from build123d import *

# Parameters (mm, degrees)
SKETCH_R              = 45
PAD_DEPTH             = 20
SKETCH001_R           = 42
POCKET_DEPTH          = 17
POCKET001_DEPTH       = 5
POLARPATTERN_COUNT    = 6
POCKET002_DEPTH       = 5
POLARPATTERN001_COUNT = 6
POCKET003_DEPTH       = 5
POLARPATTERN002_COUNT = 6
POCKET004_DEPTH       = 5
POLARPATTERN003_COUNT = 6
POCKET005_DEPTH       = 5
POLARPATTERN004_COUNT = 6
POCKET006_DEPTH       = 5
CHAMFER_SIZE2         = 2
CHAMFER_SIZE          = 5


with BuildPart() as part:
    # Sketch → Pad (new body)
    with BuildSketch(Plane.XY):
        Circle(SKETCH_R)
    extrude(amount=PAD_DEPTH)

    # Sketch001 (on Face3 of Pad) → Pocket (cut)
    with BuildSketch(Plane.XY.offset(20)):
        Circle(SKETCH001_R)
    extrude(amount=-POCKET_DEPTH, mode=Mode.SUBTRACT)

    # Sketch003 (on Face5 of Pocket) → Pocket001 (cut)
    with BuildSketch(Plane.XY.offset(3)):
        Polygon((-6.25833, 6.5), (-8.75833, 10.830127), (-13.75833, 10.830127), (-16.25833, 6.5), (-13.75833, 2.169873), (-8.75833, 2.169873), align=None)
    pocket001 = extrude(amount=-POCKET001_DEPTH, mode=Mode.SUBTRACT)

    # PolarPattern: Pocket001 ×6 about axis
    polarpattern_axis = Axis((0, 0, 3), (0, 0, 1))
    for i in range(1, POLARPATTERN_COUNT):
        add(pocket001.rotate(polarpattern_axis, i * 360 / POLARPATTERN_COUNT), mode=Mode.SUBTRACT)

    # Sketch004 (on Face41 of PolarPattern) → Pocket002 (cut)
    with BuildSketch(Plane.XY.offset(3)):
        Polygon((13.75833, -23.830127), (16.25833, -19.5), (13.75833, -15.169873), (8.75833, -15.169873), (6.25833, -19.5), (8.75833, -23.830127), align=None)
    pocket002 = extrude(amount=-POCKET002_DEPTH, mode=Mode.SUBTRACT)

    # PolarPattern001: Pocket002 ×6 about axis
    polarpattern001_axis = Axis((0, 0, 3), (0, 0, 1))
    for i in range(1, POLARPATTERN001_COUNT):
        add(pocket002.rotate(polarpattern001_axis, i * 360 / POLARPATTERN001_COUNT), mode=Mode.SUBTRACT)

    # Sketch005 (on Face77 of PolarPattern001) → Pocket003 (cut)
    with BuildSketch(Plane.XY.offset(3)):
        Polygon((2.5, -30.330127), (5, -26), (2.5, -21.669873), (-2.5, -21.669873), (-5, -26), (-2.5, -30.330127), align=None)
    pocket003 = extrude(amount=-POCKET003_DEPTH, mode=Mode.SUBTRACT)

    # PolarPattern002: Pocket003 ×6 about axis
    polarpattern002_axis = Axis((0, 0, 3), (0, 0, 1))
    for i in range(1, POLARPATTERN002_COUNT):
        add(pocket003.rotate(polarpattern002_axis, i * 360 / POLARPATTERN002_COUNT), mode=Mode.SUBTRACT)

    # Sketch006 (on Face113 of PolarPattern002) → Pocket004 (cut)
    with BuildSketch(Plane.XY.offset(3)):
        Polygon((-8.75833, -36.830127), (-6.25833, -32.5), (-8.75833, -28.169873), (-13.75833, -28.169873), (-16.25833, -32.5), (-13.75833, -36.830127), align=None)
    pocket004 = extrude(amount=-POCKET004_DEPTH, mode=Mode.SUBTRACT)

    # PolarPattern003: Pocket004 ×6 about axis
    polarpattern003_axis = Axis((0, 0, 3), (0, 0, 1))
    for i in range(1, POLARPATTERN003_COUNT):
        add(pocket004.rotate(polarpattern003_axis, i * 360 / POLARPATTERN003_COUNT), mode=Mode.SUBTRACT)

    # Sketch007 (on Face149 of PolarPattern003) → Pocket005 (cut)
    with BuildSketch(Plane.XY.offset(3)):
        Polygon((13.75833, -36.830127), (16.25833, -32.5), (13.75833, -28.169873), (8.75833, -28.169873), (6.25833, -32.5), (8.75833, -36.830127), align=None)
    pocket005 = extrude(amount=-POCKET005_DEPTH, mode=Mode.SUBTRACT)

    # PolarPattern004: Pocket005 ×6 about axis
    polarpattern004_axis = Axis((0, 0, 3), (0, 0, 1))
    for i in range(1, POLARPATTERN004_COUNT):
        add(pocket005.rotate(polarpattern004_axis, i * 360 / POLARPATTERN004_COUNT), mode=Mode.SUBTRACT)

    # Sketch008 (on Face185 of PolarPattern004) → Pocket006 (cut)
    with BuildSketch(Plane.XY.offset(3)):
        Polygon((2.5, -4.330127), (5, 0), (2.5, 4.330127), (-2.5, 4.330127), (-5, 0), (-2.5, -4.330127), align=None)
    extrude(amount=-POCKET006_DEPTH, mode=Mode.SUBTRACT)

    # Chamfer
    chamfer_edges = [part.edges().sort_by_distance(p)[0] for p in [
        (-45, 0, 20),
    ]]
    chamfer_side = part.faces().sort_by_distance((-45, 0, 10))[0]
    chamfer(chamfer_edges, length=CHAMFER_SIZE, length2=CHAMFER_SIZE2, reference=chamfer_side)


solid = part.part
Can you work these out from the model? Positions are in its coordinate system, mm. Round coordinates to 2 decimals unless told otherwise and drop trailing zeros. Order: outer loops, then holes, each group sorted by start corner. A loop starts at its lowest first (then second) coordinate and runs counter-clockwise, first axis right, second up. Notation, with made-up numbers: (12, 4) -> (16, 4) arc R36 cw to (16, 40) -> close; hole circle Ø3 at (-37.75, 63). An arc over 180 degrees is marked (long way). Write each question's results on one line, items separated by ' | '. Start each with the question number.
Item 1: If we section it at D-D, the plane z = 12.75: Write out the boundary of the cut face in (x, y).
Item 2: Please list where these lines run through material, in increasing order: L1, parallel to Y at x = 0, z = 9; L2, parallel to Z at x = -12.5, y = -39; L3, parallel to Y at x = -37, z = 9.5.
Item 3: If we section it at A-A, the plane x = 0: State how many separate pieces and enclosed holes the cut face has, then the cut area to 3 significant figures.
Item 4: Will these pins go through, and if not, where does the flat tip stop? pin 1 (3.5 mm diameter, centred on x = 23, z = 1, fed in from -Y); pin 2 (5 mm diameter, centred on x = -2, y = 11.5, fed in from +Z); pin 3 (1.5 mm diameter, centred on x = 5.5, y = 33.5, fed in from -Z); pin 4 (10 mm diameter, centred on y = -34, z = 14.5, fed in from +X).
Results:
1) outline: circle Ø90 at (0, 0); hole circle Ø84 at (0, 0)
2) L1: y = -45 to -42, 42 to 45 | L2: z = 0 to 3 | L3: y = -25.61 to -19.87, 19.87 to 25.61
3) separate pieces: 6 | enclosed holes: 0 | area: 232 mm2
4) pin 1: stops at y = -39.67 | pin 2: stops at z = 3 | pin 3: stops at z = 0 | pin 4: stops at x = 34.41
